Verification items for the finished model (mm, model axes). A direction names the side the tool comes from. Coordinates: 2 decimals unless noted, no trailing zeros. Write each loop counter-clockwise with the first axis right and the second up, starting at its lowest first coordinate (ties: lowest second). Pieces come first, ordered by that corner, then holes.
```python
from build123d import *

# Parameters (mm, degrees)
SKETCH_1_R      = 5.5
SKETCH_1_R_2    = 1.5
EXTRUDE_1_DEPTH = 2
FILLET_1_R      = 1
FILLET_2_R      = 2


with BuildPart() as part:
    # 草圖1 → 填料-伸長1 (new body)
    with BuildSketch(Plane.XY):
        Polygon((-35.75, -20.56252042), (-43, -20.56252042), (-43, -50), (-25.75, -50), (25.75, -50), (43, -50), (43, -20.56252042), (35.75, -20.56252042), (35.75, 20.56252042), (43, 20.56252042), (43, 50), (25.75, 50), (-25.75, 50), (-43, 50), (-43, 20.56252042), (-35.75, 20.56252042), align=None)
        Circle(SKETCH_1_R, mode=Mode.SUBTRACT)
        with Locations((12.5, -9)):
            Circle(SKETCH_1_R_2, mode=Mode.SUBTRACT)
        with Locations(Location((-12.5, -9, 0), (0, 0, 180))):
            Circle(SKETCH_1_R_2, mode=Mode.SUBTRACT)
        with Locations(Location((12.5, 9, 0), (0, 0, 180))):
            Circle(SKETCH_1_R_2, mode=Mode.SUBTRACT)
        with Locations((-12.5, 9)):
            Circle(SKETCH_1_R_2, mode=Mode.SUBTRACT)
        with Locations((-40, -25.5)):
            Circle(SKETCH_1_R_2, mode=Mode.SUBTRACT)
        with Locations(Location((40, -25.5, 0), (0, 0, 180))):
            Circle(SKETCH_1_R_2, mode=Mode.SUBTRACT)
        with Locations((40, 25.5)):
            Circle(SKETCH_1_R_2, mode=Mode.SUBTRACT)
        with Locations(Location((-40, 25.5, 0), (0, 0, 180))):
            Circle(SKETCH_1_R_2, mode=Mode.SUBTRACT)
        with Locations((-40, -45.5)):
            Circle(SKETCH_1_R_2, mode=Mode.SUBTRACT)
        with Locations(Location((-40, 45.5, 0), (0, 0, 180))):
            Circle(SKETCH_1_R_2, mode=Mode.SUBTRACT)
        with Locations((40, 45.5)):
            Circle(SKETCH_1_R_2, mode=Mode.SUBTRACT)
        with Locations(Location((40, -45.5, 0), (0, 0, 180))):
            Circle(SKETCH_1_R_2, mode=Mode.SUBTRACT)
        with BuildLine():
            Line((13.5, 1.5), (18.5, 1.5))
            ThreePointArc((18.5, 1.5), (20, 0), (18.5, -1.5))
            Line((18.5, -1.5), (13.5, -1.5))
            ThreePointArc((13.5, -1.5), (12, 0), (13.5, 1.5))
        make_face(mode=Mode.SUBTRACT)
        with BuildLine():
            Line((24, -8.5), (24, -21.5))
            ThreePointArc((24, -21.5), (22.5, -23), (21, -21.5))
            Line((21, -21.5), (21, -8.5))
            ThreePointArc((21, -8.5), (22.5, -7), (24, -8.5))
        make_face(mode=Mode.SUBTRACT)
        with BuildLine():
            Line((31.5, -8.5), (31.5, -21.5))
            ThreePointArc((31.5, -21.5), (30, -23), (28.5, -21.5))
            Line((28.5, -21.5), (28.5, -8.5))
            ThreePointArc((28.5, -8.5), (30, -7), (31.5, -8.5))
        make_face(mode=Mode.SUBTRACT)
        with BuildLine():
            Line((31.5, 8.5), (31.5, 21.5))
            ThreePointArc((31.5, 21.5), (30, 23), (28.5, 21.5))
            Line((28.5, 21.5), (28.5, 8.5))
            ThreePointArc((28.5, 8.5), (30, 7), (31.5, 8.5))
        make_face(mode=Mode.SUBTRACT)
        with BuildLine():
            Line((24, 8.5), (24, 21.5))
            ThreePointArc((24, 21.5), (22.5, 23), (21, 21.5))
            Line((21, 21.5), (21, 8.5))
            ThreePointArc((21, 8.5), (22.5, 7), (24, 8.5))
        make_face(mode=Mode.SUBTRACT)
        with BuildLine():
            Line((-24, 8.5), (-24, 21.5))
            ThreePointArc((-24, 21.5), (-22.5, 23), (-21, 21.5))
            Line((-21, 21.5), (-21, 8.5))
            ThreePointArc((-21, 8.5), (-22.5, 7), (-24, 8.5))
        make_face(mode=Mode.SUBTRACT)
        with BuildLine():
            Line((-31.5, 8.5), (-31.5, 21.5))
            ThreePointArc((-31.5, 21.5), (-30, 23), (-28.5, 21.5))
            Line((-28.5, 21.5), (-28.5, 8.5))
            ThreePointArc((-28.5, 8.5), (-30, 7), (-31.5, 8.5))
        make_face(mode=Mode.SUBTRACT)
        with BuildLine():
            Line((-31.5, -8.5), (-31.5, -21.5))
            ThreePointArc((-31.5, -21.5), (-30, -23), (-28.5, -21.5))
            Line((-28.5, -21.5), (-28.5, -8.5))
            ThreePointArc((-28.5, -8.5), (-30, -7), (-31.5, -8.5))
        make_face(mode=Mode.SUBTRACT)
        with BuildLine():
            Line((-24, -8.5), (-24, -21.5))
            ThreePointArc((-24, -21.5), (-22.5, -23), (-21, -21.5))
            Line((-21, -21.5), (-21, -8.5))
            ThreePointArc((-21, -8.5), (-22.5, -7), (-24, -8.5))
        make_face(mode=Mode.SUBTRACT)
        with BuildLine():
            Line((-22, -43.5), (-11, -43.5))
            ThreePointArc((-11, -43.5), (-9.5, -45), (-11, -46.5))
            Line((-11, -46.5), (-22, -46.5))
            ThreePointArc((-22, -46.5), (-23.5, -45), (-22, -43.5))
        make_face(mode=Mode.SUBTRACT)
        with BuildLine():
            Line((22, -43.5), (11, -43.5))
            ThreePointArc((11, -43.5), (9.5, -45), (11, -46.5))
            Line((11, -46.5), (22, -46.5))
            ThreePointArc((22, -46.5), (23.5, -45), (22, -43.5))
        make_face(mode=Mode.SUBTRACT)
        with BuildLine():
            Line((22, 43.5), (11, 43.5))
            ThreePointArc((11, 43.5), (9.5, 45), (11, 46.5))
            Line((11, 46.5), (22, 46.5))
            ThreePointArc((22, 46.5), (23.5, 45), (22, 43.5))
        make_face(mode=Mode.SUBTRACT)
        with BuildLine():
            Line((-22, 43.5), (-11, 43.5))
            ThreePointArc((-11, 43.5), (-9.5, 45), (-11, 46.5))
            Line((-11, 46.5), (-22, 46.5))
            ThreePointArc((-22, 46.5), (-23.5, 45), (-22, 43.5))
        make_face(mode=Mode.SUBTRACT)
        with BuildLine():
            Line((-13.5, 1.5), (-18.5, 1.5))
            ThreePointArc((-18.5, 1.5), (-20, 0), (-18.5, -1.5))
            Line((-18.5, -1.5), (-13.5, -1.5))
            ThreePointArc((-13.5, -1.5), (-12, 0), (-13.5, 1.5))
        make_face(mode=Mode.SUBTRACT)
        with BuildLine():
            Line((1.5, -23.5), (1.5, -32))
            ThreePointArc((1.5, -32), (0, -33.5), (-1.5, -32))
            Line((-1.5, -32), (-1.5, -23.5))
            ThreePointArc((-1.5, -23.5), (0, -22), (1.5, -23.5))
        make_face(mode=Mode.SUBTRACT)
        with BuildLine():
            Line((1.5, 23.5), (1.5, 32))
            ThreePointArc((1.5, 32), (0, 33.5), (-1.5, 32))
            Line((-1.5, 32), (-1.5, 23.5))
            ThreePointArc((-1.5, 23.5), (0, 22), (1.5, 23.5))
        make_face(mode=Mode.SUBTRACT)
    extrude(amount=EXTRUDE_1_DEPTH)

    # 圓角1
    fillet_1_edges = [part.edges().sort_by_distance(p)[0] for p in [
        (35.75, 20.56252042, 1),
        (35.75, -20.56252042, 1),
        (-35.75, -20.56252042, 1),
        (-35.75, 20.56252042, 1),
    ]]
    fillet(fillet_1_edges, radius=FILLET_1_R)

    # 圓角2
    fillet_2_edges = [part.edges().sort_by_distance(p)[0] for p in [
        (43, 50, 1),
        (43, 20.56252042, 1),
        (43, -20.56252042, 1),
        (43, -50, 1),
        (-43, -50, 1),
        (-43, -20.56252042, 1),
        (-43, 20.56252042, 1),
        (-43, 50, 1),
    ]]
    fillet(fillet_2_edges, radius=FILLET_2_R)


solid = part.part
```
1. Sectioned sample at A-A, the plane x = -17. Record the boundary of the cut face in (y, z), and give its area (3 significant figures).
2. Sectioned sample at B-B, the plane y = -28.5. Record the boundary of the cut face in (x, z), and give its area (3 significant figures).
3. Gauge pin test, flat ends, axial feed: P1, Ø1, axis at y = 8.5, z = 0.5, coming from the -X side; P2, Ø1, axis at y = 12.5, z = 1.5, coming from the +X side. Record the tip position at first contact, or that the pin passes through.
4. Tool access check on faces 1 (the flat face through (24, -15, 1)), 2 (the flat face through (9, 1, 0)), 3 (the cylindrical face through (-42.399, -21.133, 1.014)). Record the directions out of +Z, -Z, +X, -X, +Y, -Y that give a thin tool (end or side, any length) a straight path to the whole face; none if there is none.
5. Draft check along Y on faces 4 (the cylindrical face through (-30, 23, 1)), 5 (the flat face through (-43, 35, 1)). Enter one of: pulls with the +Y half, pulls with the -Y half, needs draft (parallel to the pull), parting line crosses it, or undercut.
6. Sectioned sample at C-C, the plane y = 0. Record the boundary of the cut face in (x, z).
7. Sectioned sample at D-D, the plane z = 0.7. Give the number of separate pieces and of enclosed holes in the cut face, and give its area (3 significant figures).
8. Material ranges on L1, parallel to Y at x = 40, z = 0.45; L2, parallel to Y at x = 30.5, z = 0.65; L3, parallel to Y at x = 12.5, z = 0.65, recorded low to high.
Outcome:
1. outline: (-50, 0) - (-46.5, 0) - (-46.5, 2) - (-50, 2) - close; (-43.5, 0) - (-1.5, 0) - (-1.5, 2) - (-43.5, 2) - close; (1.5, 0) - (43.5, 0) - (43.5, 2) - (1.5, 2) - close; (46.5, 0) - (50, 0) - (50, 2) - (46.5, 2) - close
1. area: 182 mm2
2. outline: (-43, 0) - (-1.5, 0) - (-1.5, 2) - (-43, 2) - close; (1.5, 0) - (43, 0) - (43, 2) - (1.5, 2) - close
2. area: 166 mm2
3. P1: stops at x = -35.75
3. P2: stops at x = 35.75
4. face 1: +Z, -Z
4. face 2: -Z, +X, -X, +Y, -Y
4. face 3: +Z, -Z, -X
5. face 4: undercut
5. face 5: needs draft
6. outline: (-35.75, 0) - (-20, 0) - (-20, 2) - (-35.75, 2) - close; (-12, 0) - (-5.5, 0) - (-5.5, 2) - (-12, 2) - close; (5.5, 0) - (12, 0) - (12, 2) - (5.5, 2) - close; (20, 0) - (35.75, 0) - (35.75, 2) - (20, 2) - close
7. separate pieces: 1
7. enclosed holes: 29
7. area: 7,180 mm2
8. L1: y = -50 to -47, -44 to -27, -24 to -20.56, 20.56 to 24, 27 to 44, 47 to 50
8. L2: y = -50 to -22.91, -7.09 to 7.09, 22.91 to 50
8. L3: y = -50 to -46.5, -43.5 to -10.5, -7.5 to -1.12, 1.12 to 7.5, 10.5 to 43.5, 46.5 to 50
